from build123d import *

# Parameters (mm, degrees)
CROQUIS1_R              = 72.5
SALIENTE_EXTRUIR1_DEPTH = 10
MATRIZC3_COUNT          = 6
CROQUIS13_R             = 50
SALIENTE_EXTRUIR2_DEPTH = 22


with BuildPart() as part:
    # Croquis1 → Saliente-Extruir1 (new body)
    with BuildSketch(Plane.XY):
        Circle(CROQUIS1_R)
    extrude(amount=SALIENTE_EXTRUIR1_DEPTH)

    # Croquis12 → Taladro roscado M12x1.51 (revolve, cut)
    with BuildSketch(Plane(origin=(0, 62.233623097, 0), x_dir=(0, 1, 0), z_dir=(1, 0, 0))):
        Polygon((0, 0), (0, 34.65451825), (5.25, 31.5), (5.25, 0), align=None)
    taladro_roscado_m12x1_51 = revolve(axis=Axis((0, 62.233623097, -6.35), (0, 0, 1)), mode=Mode.SUBTRACT)

    # MatrizC3: Taladro roscado M12x1.51 ×6 about axis
    matrizc3_axis = Axis((0, -0.328058282, 0), (0, 0, 1))
    for i in range(1, MATRIZC3_COUNT):
        add(taladro_roscado_m12x1_51.rotate(matrizc3_axis, i * 360 / MATRIZC3_COUNT), mode=Mode.SUBTRACT)

    # Croquis13 → Saliente-Extruir2 (add)
    with BuildSketch(Plane(origin=(0, 0, 0), x_dir=(-1, 0, 0), z_dir=(0, 0, -1))):
        Circle(CROQUIS13_R)
    extrude(amount=SALIENTE_EXTRUIR2_DEPTH)


solid = part.part
Here's how the part is built. I have some questions about the finished solid (model axes, mm). A direction names the side the tool comes from. Round coordinates to 2 decimals unless told otherwise and drop trailing zeros. Write each loop counter-clockwise with the first axis right and the second up, starting at its lowest first coordinate (ties: lowest second). Pieces come first, ordered by that corner, then holes. Notation, with made-up numbers: (66, -17.75) -> (106, -17.75) arc R21 ccw to (106, 19.25) -> close; hole circle Ø5 at (85.25, -11.5). An arc over 180 degrees is marked (long way). One line per item, written item: value.
1) If I drill on line 1 (Y direction, x = 0, z = 4); line 2 (X direction, y = 27, z = 7); line 3 (Z direction, x = 29, y = -43), over which ranges is the centre line in solid material (lowest first)? Write a range as [from, to].
Filled sheet:
line 1: y = [-72.5, -68.14], [-57.64, 56.98], [67.48, 72.5]
line 2: x = [-67.28, -57.64], [-50.72, 50.72], [57.64, 67.28]
line 3: z = [0, 10]
2) Suppose I cut it at C-C on y = 0. List the corners of the cut face in (x, z) for me.
Filled sheet:
outline: (-72.5, 0) -> (-50, 0) -> (-50, -22) -> (50, -22) -> (50, 0) -> (72.5, 0) -> (72.5, 10) -> (-72.5, 10) -> close
3) Suppose I cut it at A-A on x = 0. List the corners of the cut face in (y, z) for me.
Filled sheet:
outline: (-72.5, 0) -> (-68.14, 0) -> (-68.14, 10) -> (-72.5, 10) -> close; (-57.64, 0) -> (-50, 0) -> (-50, -22) -> (50, -22) -> (50, 0) -> (56.98, 0) -> (56.98, 10) -> (-57.64, 10) -> close; (67.48, 0) -> (72.5, 0) -> (72.5, 10) -> (67.48, 10) -> close
4) We'd pull the mould along X, two halves only. Please class faces 1 (the face through (-1, 1, 10)), 2 (the face through (2.011, 67.083, 4.93)), 3 (the face through (54.4, 36.2, 4.9)), 4 (the face through (69.15, 21.78, 4.93)): released by +X, released by -X, zero draft, split by the parting line, or undercut.
Filled sheet:
face 1: zero draft
face 2: undercut
face 3: undercut
face 4: split by the parting line
5) Suppose I cut it at D-D on z = 4. List the corners of the cut face in (x, y) for me, plus the area to 3 significant figures.
Filled sheet:
outline: circle Ø145 at (0, 0); hole circle Ø10.5 at (-54.18, -31.61); hole circle Ø10.5 at (-54.18, 30.95); hole circle Ø10.5 at (0, -62.89); hole circle Ø10.5 at (0, 62.23); hole circle Ø10.5 at (54.18, -31.61); hole circle Ø10.5 at (54.18, 30.95)
area: 16,000 mm2
6) I'm going to push flat-ended pins straight in: pin 1 Ø13.5 at (x, y) = (-54.18, 30.95) entering from +Z; pin 2 Ø10 at (y, z) = (-47.5, -14) entering from -X; pin 3 Ø9.5 at (x, y) = (0, 62.23) entering from +Z; pin 4 Ø17 at (x, y) = (0, -62.89) entering from -Z. Where does each tip first touch, or does it pass through?
Filled sheet:
pin 1: stops at z = 10
pin 2: stops at x = -26.34
pin 3: passes through
pin 4: stops at z = 0
7) Suppose I cut it at B-B on y = -32. List the corners of the cut face in (x, z) for me, plus the area to 3 significant figures.
Filled sheet:
outline: (-65.06, 0) -> (-59.42, 0) -> (-59.42, 10) -> (-65.06, 10) -> close; (-48.94, 0) -> (-38.42, 0) -> (-38.42, -22) -> (38.42, -22) -> (38.42, 0) -> (48.94, 0) -> (48.94, 10) -> (-48.94, 10) -> close; (59.42, 0) -> (65.06, 0) -> (65.06, 10) -> (59.42, 10) -> close
area: 2,780 mm2
8) For faces 5 (the face through (58.84, -29.19, 4.93)), 6 (the face through (-47.69, 15.02, -10.85)), which set-ups out of +Z, -Z, +X, -X, +Y, -Y let a thin tool reach every point of the face, with its end or its side?
Filled sheet:
face 5: +Z, -Z
face 6: -Z
